from build123d import *

# Parameters (mm, degrees)
SKETCH_1_W           = 20
SKETCH_1_H           = 28
SKETCH_1_R           = 1.6
EXTRUDE_1_DEPTH      = 5
EXTRUDE_2_DEPTH      = 5
EXTRUDE_2_DEPTH_BACK = 1.1
SKETCH_3_W           = 6.1
SKETCH_3_H           = 30.125226912
EXTRUDE_3_DEPTH      = 7
SKETCH_4_R           = 1.35
CUT_EXTRUDE_1_DEPTH  = 7
SKETCH_5_W           = 5
SKETCH_5_H           = 28
CUT_EXTRUDE_2_DEPTH  = 10
CUT_EXTRUDE_3_DEPTH  = 10


with BuildPart() as part:
    # 草图1 → 凸台-拉伸1 (new body)
    with BuildSketch(Plane(origin=(0, 0, 0), x_dir=(1, 0, 0), z_dir=(0, 1, 0))):
        Rectangle(SKETCH_1_W, SKETCH_1_H)
        with Locations(Location((-5, 10, 0), (0, 0, 270))):
            Circle(SKETCH_1_R, mode=Mode.SUBTRACT)
        with Locations(Location((-5, -10, 0), (0, 0, 90))):
            Circle(SKETCH_1_R, mode=Mode.SUBTRACT)
    extrude(amount=EXTRUDE_1_DEPTH)

    # 草图2 → 凸台-拉伸2 (add, two sides: drawn at the far end of the back side and taken through both)
    with BuildSketch(Plane(origin=(0, 0, 0), x_dir=(0, 0, -1), z_dir=(1, 0, 0)).offset(-EXTRUDE_2_DEPTH_BACK)):
        with BuildLine():
            Line((42.482395746, 143.5), (42.482395746, 113.374773088))
            add(Edge.make_bspline(
                [(10.794309538, 5), (-3.625508376, 21.700163207), (-0.038874902, 68.530494039), (24.786643579, 102.563540472), (42.482395746, 113.374773088)],
                knots=[0, 0, 0, 0, 0.510479212, 1, 1, 1, 1], degree=3))
            Line((10.794309538, 5), (-14, 5))
            add(Edge.make_bspline(
                [(-14, 5), (-21.090980053, 28.072383436), (-16.059602837, 83.599622922), (19.318940175, 126.307389699), (42.482395746, 143.5)],
                knots=[0, 0, 0, 0, 0.452386754, 1, 1, 1, 1], degree=3))
        make_face()
    extrude(amount=EXTRUDE_2_DEPTH + EXTRUDE_2_DEPTH_BACK)

    # 草图3 → 凸台-拉伸3 (add)
    with BuildSketch(Plane(origin=(0, 0, -42.482395746), x_dir=(-1, 0, 0), z_dir=(0, 0, -1))):
        with Locations((-1.95, 128.437386544)):
            Rectangle(SKETCH_3_W, SKETCH_3_H)
    extrude(amount=EXTRUDE_3_DEPTH)

    # 草图4 → 切除-拉伸1 (cut)
    with BuildSketch(Plane(origin=(5, 0, 0), x_dir=(0, 0, -1), z_dir=(1, 0, 0))):
        with Locations((45.982395746, 136.5)):
            Circle(SKETCH_4_R)
        with Locations((45.982395746, 121.5)):
            Circle(SKETCH_4_R)
    extrude(amount=-CUT_EXTRUDE_1_DEPTH, mode=Mode.SUBTRACT)

    # 草图5 → 切除-拉伸2 (cut)
    with BuildSketch(Plane(origin=(0, 5, 0), x_dir=(1, 0, 0), z_dir=(0, 1, 0))):
        with Locations((7.5, 0)):
            Rectangle(SKETCH_5_W, SKETCH_5_H)
    extrude(amount=-CUT_EXTRUDE_2_DEPTH, mode=Mode.SUBTRACT)

    # 草图6 → 切除-拉伸3 (cut)
    with BuildSketch(Plane(origin=(5, 0, 0), x_dir=(0, 0, -1), z_dir=(1, 0, 0))):
        with BuildLine():
            Line((44.782395746, 121.5), (44.782395746, 141.5))
            ThreePointArc((44.782395746, 141.5), (45.982395746, 142.7), (47.182395746, 141.5))
            Line((47.182395746, 141.5), (47.182395746, 121.5))
            ThreePointArc((47.182395746, 121.5), (45.982395746, 120.3), (44.782395746, 121.5))
        make_face()
    extrude(amount=-CUT_EXTRUDE_3_DEPTH, mode=Mode.SUBTRACT)


solid = part.part
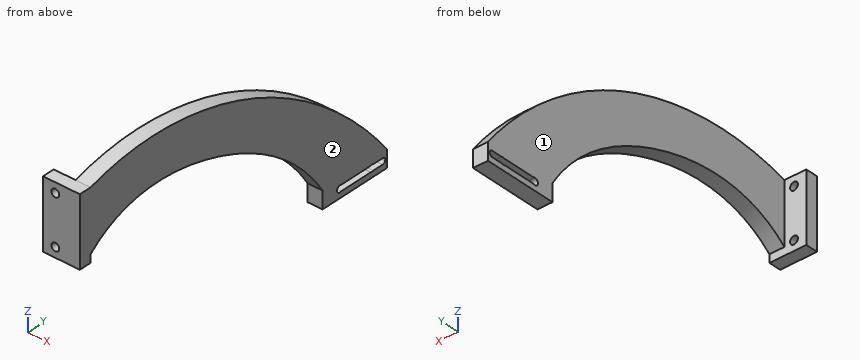
Geometry check sheet. Reference: the model listing, model coordinates, mm. Face numbers are marked on the shaded views. A direction names the side the tool comes from. Round coordinates to 2 decimals unless told otherwise and drop trailing zeros. Order: outer loops, then holes, each group sorted by start corner. A loop starts at its lowest first (then second) coordinate and runs counter-clockwise, first axis right, second up. Notation, with made-up numbers: M -13.5,77 L 32.5,77 A22 ccw 32.5,98 Z; hole C 62.5,14.25 d6. An arc over 180 degrees is marked long. Answer in a Markdown table with one row per item. Add a question column.
Item 1: Sectioned sample at A-A, the plane x = -5. Enter the section's corners in (y, z), plus the area to 3 significant figures.
Item 2: Depth check by flat-ended pin: pin 1 Ø5.5 at (x, y) = (-2.5, 3.5) entering from +Z; pin 2 Ø6.5 at (x, z) = (2, -45) entering from -Y; pin 3 Ø3 at (x, y) = (-1, 53) entering from -Z. Enter the tip coordinate at first touch or a pass-through.
Item 3: Material ranges on L1, parallel to X at y = 2.05, z = 10; L2, parallel to Y at x = -1.75, z = -7.5; L3, parallel to X at y = 75, z = 0.5, recorded low to high. Write a range as [from, to].
Item 4: Set-up check for the marked faces 1 and 2: record each of +Z, -Z, +X, -X, +Y, -Y from which the full face is reachable in a straight line by a thin tool's end or side.
Filled in:
| question | item | result |
|---|---|---|
| 1 | outline | M 0,-14 L 5,-14 L 5,-11.6 L 0,-11.6 Z; M 0,-8.4 L 5,-8.4 L 5,8.4 L 0,8.4 Z; M 0,11.6 L 5,11.6 L 5,14 L 0,14 Z |
| 1 | area | 108 mm² |
| 2 | pin 1 | stops at z = 14.26 |
| 2 | pin 2 | stops at y = 112.92 |
| 2 | pin 3 | stops at z = -2.12 |
| 3 | L1 | x = [-10, -6.6], [-3.4, 5] |
| 3 | L2 | y = [0, 5] |
| 3 | L3 | x = [-1.1, 5] |
| 4 | face 1 | +Z, -Z, -X, +Y |
| 4 | face 2 | +Z, -Z, +X, +Y, -Y |
